from build123d import *

# Parameters (mm, degrees)
PAD001_DEPTH    = 20
PAD002_DEPTH    = 5
PAD003_DEPTH    = 5
PAD_DEPTH       = 14.5
SKETCH009_R     = 10
POCKET_DEPTH    = 135.000977
SKETCH010_R     = 10
POCKET001_DEPTH = 17.001


with BuildPart() as revolution002:
    # Sketch006 → Revolution002 (revolve)
    with BuildSketch(Plane.YZ):
        Polygon((-70, 14.5), (-90, 14.5), (-87.5, 17), (-70, 17), align=None)
    revolve(axis=Axis((0, -70, 14.5), (0, 0, -1)))


with BuildPart() as revolution003:
    # Sketch007 → Revolution003 (revolve)
    with BuildSketch(Plane.YZ):
        Polygon((70, 14.5), (50, 14.5), (52.5, 17), (70, 17), align=None)
    revolve(axis=Axis((0, 70, 14.5), (0, 0, -1)))


with BuildPart() as revolution004:
    # Sketch008 → Revolution004 (revolve)
    with BuildSketch(Plane.XZ):
        Polygon((75, 14.5), (55, 14.5), (57.5, 17), (75, 17), align=None)
    revolve(axis=Axis((75, 0, 14.5), (0, 0, -1)))


with BuildPart() as pad001:
    # Sketch001 → Pad001 (new body, symmetric)
    with BuildSketch(Plane.YZ):
        Polygon((-37.5, 0), (-37.5, 70), (-22.5, 70), (-22.5, 27), (22.5, 27), (22.5, 70), (37.5, 70), (37.5, 0), align=None)
    extrude(amount=PAD001_DEPTH, both=True)


with BuildPart() as pad002:
    # Sketch002 → Pad002 (new body, symmetric)
    with BuildSketch(Plane.YZ):
        Polygon((-49.5, 14.5), (-37.5, 14.5), (-37.5, 49.5), align=None)
        Polygon((37.5, 49.5), (37.5, 14.5), (49.5, 14.5), align=None)
    extrude(amount=PAD002_DEPTH, both=True)


with BuildPart() as pad003:
    # Sketch003 → Pad003 (new body, symmetric)
    with BuildSketch(Plane.XZ):
        Polygon((20, 27), (20, 14.5), (54, 14.5), (26, 27), align=None)
    extrude(amount=PAD003_DEPTH, both=True)


with BuildPart() as revolution:
    # Sketch004 → Revolution (revolve)
    with BuildSketch(Plane.YZ):
        Polygon((-40, 87.5), (-37.5, 90), (-22.5, 90), (-20, 87.5), (-20, 70), (-40, 70), align=None)
    revolve(axis=Axis((0, -20, 70), (0, 1, 0)))


with BuildPart() as revolution001:
    # Sketch005 → Revolution001 (revolve)
    with BuildSketch(Plane.YZ):
        Polygon((20, 87.5), (22.5, 90), (37.5, 90), (40, 87.5), (40, 70), (20, 70), align=None)
    revolve(axis=Axis((0, 20, 70), (0, -1, 0)))


with BuildPart() as pocket001:
    # Sketch → Pad (new body)
    with BuildSketch(Plane.XY):
        with BuildLine():
            Line((-25, 69.999978), (-25, -70.000022))
            ThreePointArc((-25, -70.000022), (2e-05, -95.000023), (25, -69.999981))
            Line((25, -69.999981), (25, -25))
            Line((25, -25), (74.999999, -25))
            ThreePointArc((74.999999, -25), (100, 0), (75, 25))
            Line((25, 25), (75, 25))
            Line((25, 69.999981), (25, 25))
            ThreePointArc((25, 69.999981), (-2e-06, 94.999977), (-25, 69.999978))
        make_face()
    extrude(amount=PAD_DEPTH)

    # Fusion: union Revolution002, Revolution003, Revolution004, Pad001, Pad002, Pad003, Revolution, Revolution001
    add(revolution002.part)
    add(revolution003.part)
    add(revolution004.part)
    add(pad001.part)
    add(pad002.part)
    add(pad003.part)
    add(revolution.part)
    add(revolution001.part)

    # Sketch009 (on Face42 of Fusion) → Pocket (cut, through all)
    with BuildSketch(Plane.XZ.offset(40)):
        with Locations((0, 70)):
            Circle(SKETCH009_R)
    extrude(amount=-POCKET_DEPTH, mode=Mode.SUBTRACT)

    # Sketch010 (on Face42 of Pocket) → Pocket001 (cut, through all)
    with BuildSketch(Plane.XY.offset(17)):
        with Locations((0, -70)):
            Circle(SKETCH010_R)
        with Locations((75, 0)):
            Circle(SKETCH010_R)
        with Locations((0, 70)):
            Circle(SKETCH010_R)
    extrude(amount=-POCKET001_DEPTH, mode=Mode.SUBTRACT)


solid = pocket001.part
For this review, take the finished solid that the model builds, in its own axes (mm). A direction names the side the tool comes from. Give positions to 0.01 mm unless a question says otherwise; leave off trailing zeros. Order: outer loops, then holes, each group sorted by start corner. A loop starts at its lowest first (then second) coordinate and runs counter-clockwise, first axis right, second up. Notation, with made-up numbers: (74.5, 87.25) - (122.5, 87.25) arc R18 cw to (122.5, 100.25) - close; hole circle Ø5 at (16.5, -25.5). An arc over 180 degrees is marked (long way). Answer as a JSON object with one key per item and string values. Group by question number.
Item 1: Clearance check with flat-ended pins moving along their axes: pin 1 Ø20 at (x, z) = (-1.5, 53.5) entering from -Y; pin 2 Ø5 at (x, y) = (23.5, 58.5) entering from +Z; pin 3 Ø20 at (x, z) = (2, 46) entering from -Y; pin 4 Ø12 at (x, y) = (37.5, 23.5) entering from -Z. State where each tip first meets the part, or that it passes through.
Item 2: Wall thickness on line 1 along Y through (x, z) = (7.5, 62); line 2 along Z through (x, y) = (0, 29); line 3 along Y through (x, z) = (19.5, 55): over which ranges is each line inside the solid? List them lowest first.
Item 3: Machinability: for faces 1 (the flat face through (40.2, -0.07, 20.66)), 2 (the flat face through (50, -25, 7)), 3 (the flat face through (-8, -20, 78)), 4 (the flat face through (8, 62, 17)), which of the approach directions +Z, -Z, +X, -X, +Y, -Y give a long, thin tool a straight path to every point of the face, cutting with its end or side? Answer none if there is none.
Item 4: Take a section at C-C on x = 33. Give the boundary of the cut face in (y, z) (3 decimals).
Item 5: Draft analysis for pull direction Y (two halves, no side actions). For faces 5 (the flat face through (8, -78, 17)), 6 (the conical face through (-6.749, -20.121, 86.278)), 7 (the flat face through (50, 25, 7)), state which applies: pulls with the +Y half, pulls with the -Y half, needs draft (parallel to the pull), parting line crosses it, or undercut.
Item 6: Take a section at A-A on y = 0. Give the boundary of the cut face in (x, z), and give its area (3 significant figures).
Item 7: Take a section at D-D on z = 19. Give the boundary of the cut face in (x, y).
Item 8: Take a section at B-B on z = 8. Give the boundary of the cut face in (x, y).
Reported:
{
 "1": {"pin 1": "y = -40", "pin 2": "z = 14.5", "pin 3": "y = -42.13", "pin 4": "z = 0"},
 "2": {"line 1": "-40 to -20, 20 to 40", "line 2": "0 to 60, 80 to 90", "line 3": "-37.5 to -22.5, 22.5 to 37.5"},
 "3": {"face 1": "+Z, +Y, -Y", "face 2": "+Z, -Z, +X, -Y", "face 3": "+Z, +X, -X", "face 4": "+Z, +X, -X, +Y"},
 "4": {"outline": "(-25, 0) - (25, 0) - (25, 14.5) - (5, 14.5) - (5, 23.875) - (-5, 23.875) - (-5, 14.5) - (-25, 14.5) - close"},
 "5": {"face 5": "needs draft", "face 6": "undercut", "face 7": "pulls with the +Y half"},
 "6": {"outline": "(-25, 0) - (65, 0) - (65, 17) - (57.5, 17) - (55, 14.5) - (54, 14.5) - (26, 27) - (-20, 27) - (-20, 14.5) - (-25, 14.5) - close; (85, 0) - (100, 0) - (100, 14.5) - (95, 14.5) - (92.5, 17) - (85, 17) - close", "area": "2,320 mm^2"},
 "7": {"outline": "(-20, -37.5) - (-5, -37.5) - (-5, -47.96) - (5, -47.96) - (5, -37.5) - (20, -37.5) - (20, -5) - (43.92, -5) - (43.92, 5) - (20, 5) - (20, 37.5) - (5, 37.5) - (5, 47.96) - (-5, 47.96) - (-5, 37.5) - (-20, 37.5) - close"},
 "8": {"outline": "(-25, -70) arc R25 ccw to (25, -70) - (25, -25) - (75, -25) arc R25 ccw to (75, 25) - (25, 25) - (25, 70) arc R25 ccw to (-25, 70) - close; hole circle Ø20 at (0, -70); hole circle Ø20 at (0, 70); hole circle Ø20 at (75, 0)"}
}
